```python
from build123d import *

# Parameters (mm, degrees)
F0_W      = 40
F0_H      = 25
F1_DEPTH  = 5
F4_W      = 6
F4_H      = 6
F5_DEPTH  = 1
F3_W      = 6
F3_H      = 6
F6_DEPTH  = 1
F7_R      = 2.99999
F8_R      = 1.5
F9_DEPTH  = 30
F10_DEPTH = 10


# Not quite as in the source:
# - a fillet or chamfer is up to 0.001 mm smaller than in the source, because OpenCascade refuses the exact size


with BuildPart() as f1:
    # F0 (on Top) → F1 (new body)
    with BuildSketch(Plane.XY):
        Rectangle(F0_W, F0_H)
    extrude(amount=F1_DEPTH)

    # F4 (on face) → F5 (join)
    with BuildSketch(Plane.XZ.offset(12.5)):
        with Locations((9, 8)):
            Rectangle(F4_W, F4_H)
    extrude(amount=-F5_DEPTH)

    # F3 (on face) → F6 (join)
    with BuildSketch(Plane(origin=(0, 12.5, 0), x_dir=(-1, 0, 0), z_dir=(0, 1, 0))):
        with Locations((-9, 8)):
            Rectangle(F3_W, F3_H)
    extrude(amount=-F6_DEPTH)

    # F7 (radius 3 in the source; OpenCascade refuses exactly that, so slightly less here)
    f7_edges = [f1.edges().sort_by_distance(p)[0] for p in [
        (6, 12, 11),
        (12, 12, 11),
        (6, -12, 11),
        (12, -12, 11),
    ]]
    fillet(f7_edges, radius=F7_R)

    # F8 (on face) → F9 (cut)
    with BuildSketch(Plane(origin=(0, 12.5, 0), x_dir=(-1, 0, 0), z_dir=(0, 1, 0))):
        with Locations((-9, 8)):
            Circle(F8_R)
    extrude(amount=-F9_DEPTH, mode=Mode.SUBTRACT)

    # F10 (add): a face of the model
    f10_faces = [f1.faces().sort_by_distance(p)[0] for p in [
        (20, 0, 2.5),
    ]]
    extrude(f10_faces, amount=F10_DEPTH)


solid = f1.part
```
The model under review builds one solid part; all positions refer to its coordinate system, in mm. A direction names the side the tool comes from. Round coordinates to 2 decimals unless told otherwise and drop trailing zeros. Order: outer loops, then holes, each group sorted by start corner. A loop starts at its lowest first (then second) coordinate and runs counter-clockwise, first axis right, second up.
Item 1: Machinability: for faces 1 (the cylindrical face through (10.2, -12, 7.1)), 2 (the flat face through (9, 11.5, 6)), 3 (the flat face through (6, 12, 6)), 4 (the flat face through (12, -12, 6)), which of the approach directions +Z, -Z, +X, -X, +Y, -Y give a long, thin tool a straight path to every point of the face, cutting with its end or side? Answer none if there is none.
Working result:
face 1: +Y, -Y
face 2: +Z, +X, -X
face 3: +Z, -X, +Y, -Y
face 4: +Z, +X, +Y, -Y
Item 2: For pin 1 (1 mm diameter, centred on x = 23.5, y = 0, fed in from -Z); pin 2 (1.1 mm diameter, centred on y = 12, z = 6, fed in from -X); pin 3 (1.1 mm diameter, centred on y = 12, z = 6, fed in from +X); pin 4 (7.5 mm diameter, centred on x = 2.5, y = -2.5, fed in from +Z), all flat-tipped, find the tip position at first contact; note any pin that passes through.
Working result:
pin 1: stops at z = 0
pin 2: stops at x = 6
pin 3: stops at x = 12
pin 4: stops at z = 5
Item 3: Add section C-C, the plane x = 19. State the section outline as (y, z) points.
Working result:
outline: (-12.5, 0) - (12.5, 0) - (12.5, 5) - (-12.5, 5) - close
Item 4: Add section A-A, the plane z = 10.25. State the section outline as (x, y) points.
Working result:
outline: (7.02, -12.5) - (10.98, -12.5) - (10.98, -11.5) - (7.02, -11.5) - close; (7.02, 11.5) - (10.98, 11.5) - (10.98, 12.5) - (7.02, 12.5) - close
Item 5: Add section B-B, the plane y = 0. State the section outline as (x, z) points, and give its area (3 significant figures).
Working result:
outline: (-20, 0) - (30, 0) - (30, 5) - (-20, 5) - close
area: 250 mm2
Item 6: Draft analysis for pull direction Y (two halves, no side actions). For faces 5 (the flat face through (9, -11.5, 6)), 6 (the flat face through (30, 0, 2)), 7 (the flat face through (5, 12.5, 3)), state which applies: released by +Y, released by -Y, zero draft, split by the parting line, or undercut.
Working result:
face 5: undercut
face 6: zero draft
face 7: released by +Y
Item 7: To check wall thickness, follow probe 1 along Z at (x, y) = (9, 12.1); probe 2 along Y at (x, z) = (7, 8.25); probe 3 along Z at (x, y) = (-2, 9). State the ranges of each line that lie inside material, in increasing order.
Working result:
probe 1: z = 0 to 6.5, 9.5 to 11
probe 2: y = -12.5 to -11.5, 11.5 to 12.5
probe 3: z = 0 to 5
